Model file for the job. Use its own axes, mm. Coordinates: 2 decimals unless noted, no trailing zeros. Loops run counter-clockwise (first coordinate to the right, second up) from the corner with the lowest first, then second, coordinate; pieces in that order, holes last. Notation, with made-up numbers: M -6.5,46 L 22.5,46 A18 ccw 22.5,67 Z; hole C -5,18.25 d5. An arc over 180 degrees is marked long. One line per question, with ' | ' between items. Start each with the question number.
```python
from build123d import *

# Parameters (mm, degrees)
SKETCH1_R           = 6.4135
SKETCH1_R_2         = 2.413
SKETCH1_R_3         = 6.35
BOSS_EXTRUDE1_DEPTH = 6.35
FILLET1_R           = 5.08


with BuildPart() as part:
    # Sketch1 → Boss-Extrude1 (new body)
    with BuildSketch(Plane.XY):
        with BuildLine():
            Line((273.05, 36.83), (273.05, 29.21))
            ThreePointArc((273.05, 29.21), (270.074204897, 22.025795103), (262.89, 19.05))
            Line((262.89, 19.05), (-19.05, 19.05))
            Line((-19.05, 19.05), (-19.05, -19.05))
            Line((-19.05, -19.05), (285.190051277, -19.05))
            Line((285.190051277, -19.05), (288.29, -19.05))
            ThreePointArc((288.29, -19.05), (304.454461018, -12.354461018), (311.15, 3.81))
            Line((311.15, 3.81), (311.15, 36.83))
            Line((311.15, 36.83), (273.05, 36.83))
        make_face()
        Circle(SKETCH1_R, mode=Mode.SUBTRACT)
        with Locations((0, 11.43)):
            Circle(SKETCH1_R_2, mode=Mode.SUBTRACT)
        with Locations((11.43, 0)):
            Circle(SKETCH1_R_2, mode=Mode.SUBTRACT)
        with Locations((0, -11.43)):
            Circle(SKETCH1_R_2, mode=Mode.SUBTRACT)
        with Locations((-11.43, 0)):
            Circle(SKETCH1_R_2, mode=Mode.SUBTRACT)
        with Locations((292.1, 20.066)):
            Circle(SKETCH1_R_3, mode=Mode.SUBTRACT)
    extrude(amount=BOSS_EXTRUDE1_DEPTH)

    # Fillet1
    fillet1_edges = [part.edges().sort_by_distance(p)[0] for p in [
        (311.15, 36.83, 3.175),
    ]]
    fillet(fillet1_edges, radius=FILLET1_R)


solid = part.part
```
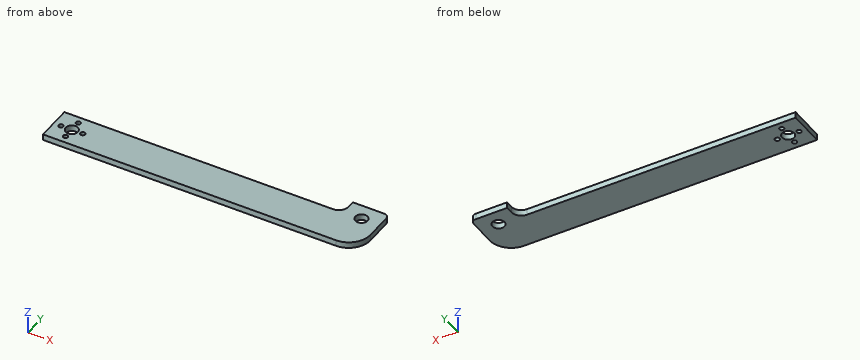
(1) Pin check, flat tips, straight feed: P1, Ø12, axis at x = 247.5, y = 27, coming from the -Z side; P2, Ø1, axis at x = 166.5, z = 4, coming from the +Y side. Stop position of each tip, or through.
(2) Band-saw the part on C-C on x = 104.5. Write the cut outline in (y, z), then the cut area to 3 significant figures.
(3) Band-saw the part on B-B on z = 2. Write the cut outline in (x, y), then the cut area to 3 significant figures.
(4) Drill centre lines: line 1 (Y direction, x = 0, z = 4.5); line 2 (X direction, y = -1.5, z = 3.75); line 3 (Y direction, x = 11.43, z = 3). Where is each one in solid material? Low to high. Write a range as [from, to].
(5) Band-saw the part on A-A on x = 292.1. Write the cut outline in (y, z), then the cut area to 3 significant figures.
Computed values:
1) P1: through | P2: y = 19.05
2) outline: M -19.05,0 L 19.05,0 L 19.05,6.35 L -19.05,6.35 Z | area: 242 mm^2
3) outline: M -19.05,-19.05 L 288.29,-19.05 A22.86 ccw 311.15,3.81 L 311.15,31.75 A5.08 ccw 306.07,36.83 L 273.05,36.83 L 273.05,29.21 A10.16 cw 262.89,19.05 L -19.05,19.05 Z; hole C -11.43,0 d4.83; hole C 0,0 d12.83; hole C 0,-11.43 d4.83; hole C 0,11.43 d4.83; hole C 11.43,0 d4.83; hole C 292.1,20.07 d12.7 | area: 12,800 mm^2
4) line 1: [-19.05, -13.84], [-9.02, -6.41], [6.41, 9.02], [13.84, 19.05] | line 2: [-19.05, -13.32], [-9.54, -6.24], [6.24, 9.54], [13.32, 310.52] | line 3: [-19.05, -2.41], [2.41, 19.05]
5) outline: M -18.73,0 L 13.72,0 L 13.72,6.35 L -18.73,6.35 Z; M 26.42,0 L 36.83,0 L 36.83,6.35 L 26.42,6.35 Z | area: 272 mm^2
